```python
from build123d import *

# Parameters (mm, degrees)
F0_W      = 25.4
F0_H      = 31.75
F1_DEPTH  = 50.8
F2_R      = 14.351
F3_DEPTH  = 101.6
F4_W      = 12.7
F4_H      = 19.05
F5_DEPTH  = 254
F6_W      = 12.7
F6_H      = 19.05
F7_DEPTH  = 127
F9_DEPTH  = 6.35
F11_DEPTH = 6.35
F13_DEPTH = 50.8
F15_DEPTH = 558.8
F16_R     = 25.39999


# Not quite as in the source:
# - a fillet or chamfer is up to 0.001 mm smaller than in the source, because OpenCascade refuses the exact size


with BuildPart() as f1:
    # F0 (on Front) → F1 (new body)
    with BuildSketch(Plane.XZ):
        Polygon((0, 19.05), (0, 0), (139.7, 0), (139.7, 19.05), (95.25, 19.05), (69.85, 19.05), (44.45, 19.05), align=None)
        with Locations((57.15, 34.925)):
            Rectangle(F0_W, F0_H)
        with Locations((82.55, 34.925)):
            Rectangle(F0_W, F0_H)
    extrude(amount=F1_DEPTH)

    # F2 (on face) → F3 (cut)
    with BuildSketch(Plane.XY.offset(50.8)):
        with Locations((69.85, -25.4)):
            Circle(F2_R)
    extrude(amount=-F3_DEPTH, mode=Mode.SUBTRACT)

    # F4 (on face) → F5 (cut)
    with BuildSketch(Plane.XZ.offset(50.8)):
        with Locations((69.85, 41.275)):
            Rectangle(F4_W, F4_H)
    extrude(amount=-F5_DEPTH, mode=Mode.SUBTRACT)

    # F6 (on face) → F7 (cut)
    with BuildSketch(Plane.YZ.offset(95.25)):
        with Locations((-25.4, 41.275)):
            Rectangle(F6_W, F6_H)
    extrude(amount=-F7_DEPTH, mode=Mode.SUBTRACT)

    # F8 (on face) → F9 (cut)
    with BuildSketch(Plane.XY.offset(19.05)):
        with BuildLine():
            ThreePointArc((114.3, -36.576), (122.2026253865, -33.3026253865), (125.476, -25.4))
            ThreePointArc((125.476, -25.4), (106.3973746135, -17.4973746135), (114.3, -36.576))
        make_face()
    extrude(amount=-F9_DEPTH, mode=Mode.SUBTRACT)

    # F10 (on face) → F11 (cut)
    with BuildSketch(Plane.XY.offset(19.05)):
        with BuildLine():
            ThreePointArc((25.4, -36.576), (33.3026253865, -33.3026253865), (36.576, -25.4))
            ThreePointArc((36.576, -25.4), (17.4973746135, -17.4973746135), (25.4, -36.576))
        make_face()
    extrude(amount=-F11_DEPTH, mode=Mode.SUBTRACT)

    # F12 (on face) → F13 (cut)
    with BuildSketch(Plane(origin=(0, 0, 0), x_dir=(1, 0, 0), z_dir=(0, 0, -1))):
        with BuildLine():
            ThreePointArc((25.4, 19.05), (29.8901280605, 20.9098719395), (31.75, 25.4))
            ThreePointArc((31.75, 25.4), (20.9098719395, 29.8901280605), (25.4, 19.05))
        make_face()
    extrude(amount=-F13_DEPTH, mode=Mode.SUBTRACT)

    # F14 (on face) → F15 (cut)
    with BuildSketch(Plane(origin=(0, 0, 0), x_dir=(1, 0, 0), z_dir=(0, 0, -1))):
        with BuildLine():
            ThreePointArc((114.3, 19.05), (118.7901280605, 20.9098719395), (120.65, 25.4))
            ThreePointArc((120.65, 25.4), (109.8098719395, 29.8901280605), (114.3, 19.05))
        make_face()
    extrude(amount=-F15_DEPTH, mode=Mode.SUBTRACT)

    # F16 (radius 25.4 in the source; OpenCascade refuses exactly that, so slightly less here)
    f16_edges = [f1.edges().sort_by_distance(p)[0] for p in [
        (95.25, 0, 34.925),
        (95.25, -50.8, 34.925),
        (44.45, 0, 34.925),
        (44.45, -50.8, 34.925),
        (0, -50.8, 9.525),
        (0, 0, 9.525),
        (139.7, -50.8, 9.525),
        (139.7, 0, 9.525),
    ]]
    fillet(f16_edges, radius=F16_R)


solid = f1.part
```
Read the model definition and answer for the solid it produces. Units are mm, in the model's axes. A direction names the side the tool comes from. Coordinates: 2 decimals unless noted, no trailing zeros. Loops run counter-clockwise (first coordinate to the right, second up) from the corner with the lowest first, then second, coordinate; pieces in that order, holes last. Notation, with made-up numbers: (29, 21.5) - (82, 21.5) arc R25 ccw to (82, 39.5) - close; hole circle Ø6 at (25.25, 5.5). An arc over 180 degrees is marked (long way). Answer in a Markdown table with one row per item.
1. Find section A-A, the plane z = 35.5. Write down the section's boundary in (x, y), then the cut area to 3 significant figures.
Conclusion:
| item | result |
|---|---|
| outline | (45.26, -31.75) arc R25.4 ccw to (63.5, -49.99) - (63.5, -38.27) arc R14.35 cw to (56.98, -31.75) - close; (45.26, -19.05) - (56.98, -19.05) arc R14.35 cw to (63.5, -12.53) - (63.5, -0.81) arc R25.4 ccw to start; (76.2, -49.99) arc R25.4 ccw to (94.44, -31.75) - (82.72, -31.75) arc R14.35 cw to (76.2, -38.27) - close; (76.2, -12.53) arc R14.35 cw to (82.72, -19.05) - (94.44, -19.05) arc R25.4 ccw to (76.2, -0.81) - close |
| area | 808 mm² |
2. Which of the six approach directions +Z, -Z, +X, -X, +Y, -Y give full straight-line access (tool end or side, diameter ignored) to faces 1 (the face through (76.2, -44, 41)), 2 (the face through (30, -30, 12.7)), 3 (the face through (87.61, -43.56, 35.15)), 4 (the face through (132.06, -7.24, 9.66)), 5 (the face through (51, -19.05, 41))?
Conclusion:
| item | result |
|---|---|
| face 1 | +Z, +Y, -Y |
| face 2 | +Z |
| face 3 | +Z, +X, -Y |
| face 4 | +Z, -Z, +X, +Y |
| face 5 | +Z, +X, -X |
3. Given pin 1 (9.5 mm diameter, centred on y = -44, z = 40.5, fed in from -X); pin 2 (6 mm diameter, centred on x = 48.5, z = 43, fed in from -Y); pin 3 (9.5 mm diameter, centred on x = 87, z = 38.5, fed in from +Y), each flat-ended and moving along its own axis, determine where each tip first touches the part or whether it passes through.
Conclusion:
| item | result |
|---|---|
| pin 1 | stops at x = 48.56 |
| pin 2 | stops at y = -42.96 |
| pin 3 | stops at y = -3.23 |
4. Find section B-B, the plane x = 111.5. Write down the section's boundary in (y, z), then the cut area to 3 significant figures.
Conclusion:
| item | result |
|---|---|
| outline | (-50.8, 0) - (-31.1, 0) - (-31.1, 12.7) - (-36.22, 12.7) - (-36.22, 19.05) - (-50.8, 19.05) - close; (-19.7, 0) - (0, 0) - (0, 19.05) - (-14.58, 19.05) - (-14.58, 12.7) - (-19.7, 12.7) - close |
| area | 686 mm² |
5. Determine the mould class of faces 6 (the face through (57, -39, 50.8)), 7 (the face through (52.09, -43.56, 35.15)), 8 (the face through (51, -31.75, 41)) for opening direction Y: +Y half, -Y half, draft (parallel to the pull), parting line (faces both ways), or undercut.
Conclusion:
| item | result |
|---|---|
| face 6 | draft |
| face 7 | -Y half |
| face 8 | undercut |
6. Find section D-D, the plane y = -17. Write down the section's boundary in (x, z), then the cut area to 3 significant figures.
Conclusion:
| item | result |
|---|---|
| outline | (1.43, 0) - (58.21, 0) - (58.21, 50.8) - (45.88, 50.8) - (45.88, 19.05) - (32.77, 19.05) - (32.77, 12.7) - (18.03, 12.7) - (18.03, 19.05) - (1.43, 19.05) - close; (81.49, 0) - (138.27, 0) - (138.27, 19.05) - (121.67, 19.05) - (121.67, 12.7) - (106.93, 12.7) - (106.93, 19.05) - (93.82, 19.05) - (93.82, 50.8) - (81.49, 50.8) - close |
| area | 2,760 mm² |
7. Straight lines are drawn through the part: line 1 (X direction, y = -25, z = 15); line 2 (X direction, y = -25, z = 4); line 3 (Y direction, x = 25.4, z = 4.5). For each, find the intervals that lie inside material, in ascending order.
Conclusion:
| item | result |
|---|---|
| line 1 | x = 0 to 14.23, 36.57 to 55.5, 84.2 to 103.13, 125.47 to 139.7 |
| line 2 | x = 0 to 19.06, 31.74 to 55.5, 84.2 to 107.96, 120.64 to 139.7 |
| line 3 | y = -50.8 to -31.75, -19.05 to 0 |
